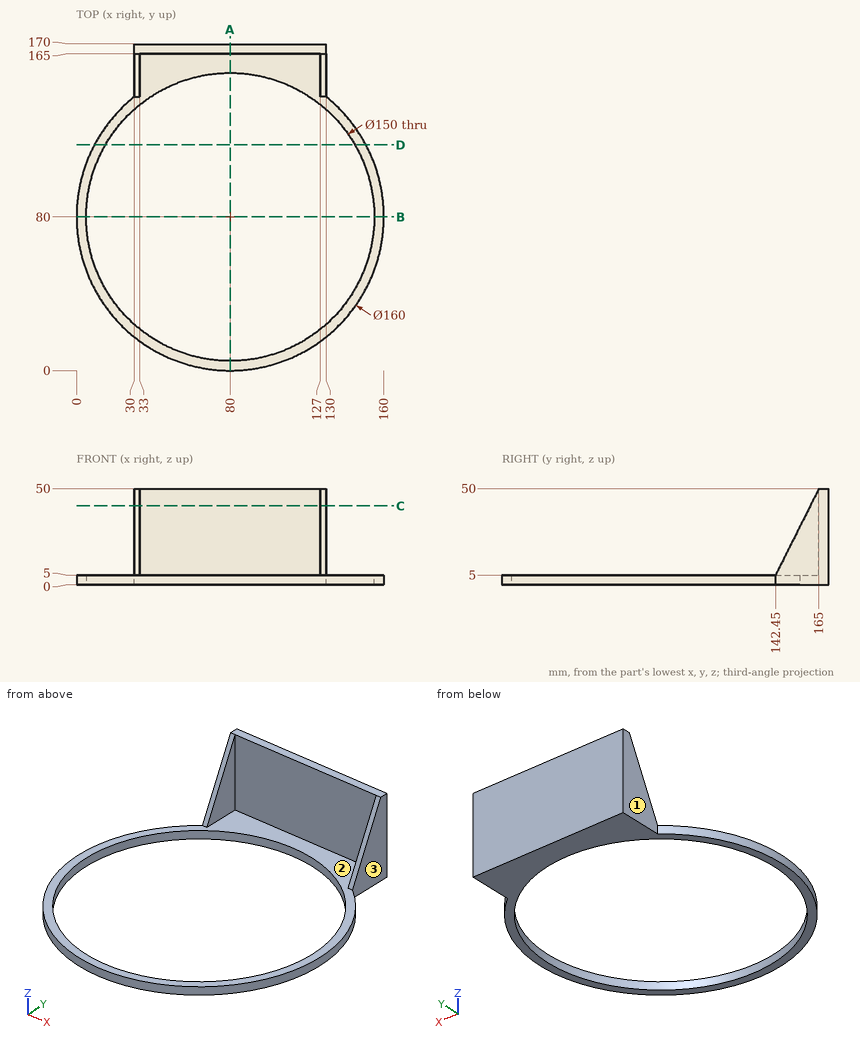
Geometry check sheet. Reference: drawing and pictorial views, mm from the part's lowest x, y, z. A direction names the side the tool comes from. Give positions to 0.01 mm unless a question says otherwise; leave off trailing zeros. Loops run counter-clockwise (first coordinate to the right, second up) from the corner with the lowest first, then second, coordinate; pieces in that order, holes last. Notation, with made-up numbers: (-37.75, -14.75) -> (-14.75, -14.75) arc R27 ccw to (-14.75, 12.25) -> close; hole circle Ø8 at (60.5, 38.5). An arc over 180 degrees is marked (long way). Answer in a Markdown table with one row per item. Add a question column.
1) Material ranges on probe 1 along X at (y, z) = (80, 1.4); probe 2 along Y at (x, z) = (80, 3.5); probe 3 along X at (y, z) = (161, 25.5), recorded low to high. Write a range as from..to.
2) Cross-section at D-D on y = 117.5. Record the boundary of the cut face in (x, z).
3) Cross-section at A-A on x = 80. Record the boundary of the cut face in (y, z), and give its area (3 significant figures).
4) Cross-section at C-C on z = 41. Record the boundary of the cut face in (x, y), and give its area (3 significant figures).
5) Set-up check for the marked faces 1, 2 and 3: record each of +Z, -Z, +X, -X, +Y, -Y from which the full face is reachable in a straight line by a thin tool's end or side.
6) Gauge pin test, flat ends, axial feed: P1, Ø25, axis at y = 155.5, z = 32.5, coming from the +X side; P2, Ø13.5, axis at x = 101, z = 19, coming from the -Y side; P3, Ø7, axis at y = 157.5, z = 25.5, coming from the -X side. Record the tip position at first contact, or that the pin passes through.
7) Cross-section at B-B on y = 80. Record the boundary of the cut face in (x, z).
Outcome:
| question | item | result |
|---|---|---|
| 1 | probe 1 | x = 0..5, 155..160 |
| 1 | probe 2 | y = 0..5, 155..170 |
| 1 | probe 3 | x = 30..33, 127..130 |
| 2 | outline | (9.33, 0) -> (15.05, 0) -> (15.05, 5) -> (9.33, 5) -> close; (144.95, 0) -> (150.67, 0) -> (150.67, 5) -> (144.95, 5) -> close |
| 3 | outline | (0, 0) -> (5, 0) -> (5, 5) -> (0, 5) -> close; (155, 0) -> (170, 0) -> (170, 50) -> (165, 50) -> (165, 5) -> (155, 5) -> close |
| 3 | area | 325 mm^2 |
| 4 | outline | (30, 160.49) -> (33, 160.49) -> (33, 165) -> (127, 165) -> (127, 160.49) -> (130, 160.49) -> (130, 170) -> (30, 170) -> close |
| 4 | area | 527 mm^2 |
| 5 | face 1 | +Z, -Z, -X, +Y |
| 5 | face 2 | +Z, -Y |
| 5 | face 3 | +Z, -Z, +X, +Y |
| 6 | P1 | stops at x = 130 |
| 6 | P2 | stops at y = 165 |
| 6 | P3 | stops at x = 30 |
| 7 | outline | (0, 0) -> (5, 0) -> (5, 5) -> (0, 5) -> close; (155, 0) -> (160, 0) -> (160, 5) -> (155, 5) -> close |
